from build123d import *

# Parameters (mm, degrees)
ESQUISSE2_R             = 1
ENL_V_MAT_EXTRU_1_DEPTH = 2.6
ESQUISSE3_R             = 1.75
ENL_V_MAT_EXTRU_2_DEPTH = 1.1


with BuildPart() as part:
    # Esquisse1 → Révolution1 (revolve)
    with BuildSketch(Plane(origin=(0, 0, 0), x_dir=(0, 0, -1), z_dir=(1, 0, 0)), mode=Mode.PRIVATE) as r_volution1_sk:
        Polygon((-13.5, 0), (-13.5, 1.15), (-15.6, 1.15), (-15.6, 0), (-20.5, 0), (-20.5, -0.6), (-19.75, -1.6), (-13.1, -1.6), (-13.1, -0.6), (-12.5, -0.6), (-12.5, 0), align=None)
    revolve(r_volution1_sk.sketch.rotate(Axis((0, -40.878639624, 0), (0, 1, 0)), 180), axis=Axis((0, -40.878639624, 0), (0, 1, 0)))  # turned: the seam where the file's is

    # Esquisse2 → Enlèv. mat.-Extru.1 (cut, through all)
    with BuildSketch(Plane(origin=(0, 0, 0), x_dir=(1, 0, 0), z_dir=(0, 1, 0))):
        with Locations(Location((0, -18.4, 0), (0, 0, 270))):  # turned: the seam where the file's is
            Circle(ESQUISSE2_R)
        with Locations(Location((17.4994399, -5.685912696, 0), (0, 0, 270))):  # turned: the seam where the file's is
            Circle(ESQUISSE2_R)
        with Locations(Location((10.815248642, 14.885912696, 0), (0, 0, 270))):  # turned: the seam where the file's is
            Circle(ESQUISSE2_R)
        with Locations(Location((-10.815248642, 14.885912696, 0), (0, 0, 270))):  # turned: the seam where the file's is
            Circle(ESQUISSE2_R)
        with Locations(Location((-17.4994399, -5.685912696, 0), (0, 0, 270))):  # turned: the seam where the file's is
            Circle(ESQUISSE2_R)
    extrude(amount=-ENL_V_MAT_EXTRU_1_DEPTH, mode=Mode.SUBTRACT)

    # Esquisse3 → Enlèv. mat.-Extru.2 (cut)
    with BuildSketch(Plane.XZ.offset(1.6)):
        with Locations(Location((0, 18.4, 0), (0, 0, 270))):  # turned: the seam where the file's is
            Circle(ESQUISSE3_R)
        with Locations(Location((17.4994399, 5.685912696, 0), (0, 0, 270))):  # turned: the seam where the file's is
            Circle(ESQUISSE3_R)
        with Locations(Location((10.815248642, -14.885912696, 0), (0, 0, 270))):  # turned: the seam where the file's is
            Circle(ESQUISSE3_R)
        with Locations(Location((-10.815248642, -14.885912696, 0), (0, 0, 270))):  # turned: the seam where the file's is
            Circle(ESQUISSE3_R)
        with Locations(Location((-17.4994399, 5.685912696, 0), (0, 0, 270))):  # turned: the seam where the file's is
            Circle(ESQUISSE3_R)
    extrude(amount=-ENL_V_MAT_EXTRU_2_DEPTH, mode=Mode.SUBTRACT)


solid = part.part
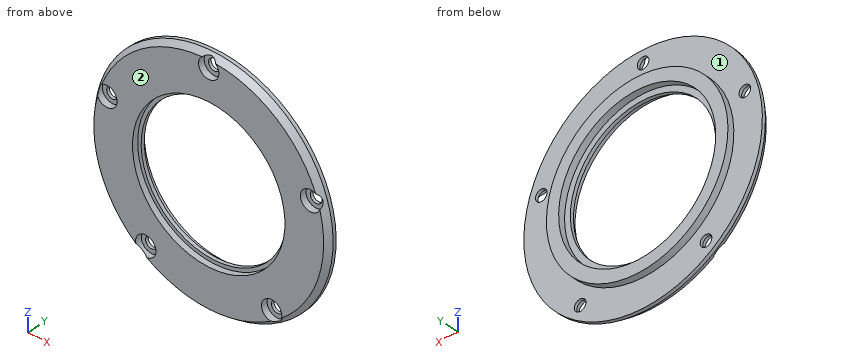
Verification items for the finished model (mm, model axes). Face numbers are marked on the shaded views. A direction names the side the tool comes from. Coordinates: 2 decimals unless noted, no trailing zeros. Order: outer loops, then holes, each group sorted by start corner. A loop starts at its lowest first (then second) coordinate and runs counter-clockwise, first axis right, second up. Notation, with made-up numbers: (-31.5, 63) -> (-10.5, 63) arc R26 cw to (-10.5, 80) -> close; hole circle Ø4 at (64, -26). An arc over 180 degrees is marked (long way). Use CSV: the item, a comma, the result in double quotes. Start each with the question number.
Q1. Section check A-A, the plane z = 0. Record the cut outline in (x, y).
Q2. Depth check by flat-ended pin: P1, Ø3, axis at x = -17.5, z = 5.69, coming from the +Y side; P2, Ø1.5, axis at y = -1, z = 8, coming from the +X side; P3, Ø1, axis at x = 18, z = 5, coming from the -Y side. Enter the tip coordinate at first touch or a pass-through.
Q3. Section check B-B, the plane x = 0. Give the number of separate pieces and of enclosed holes in the cut face, and give its area (3 significant figures).
Q4. Section check C-C, the plane y = 0.65. Record the cut outline in (x, z), and give its area (3 significant figures).
Q5. Tool access check on the marked faces 1 and 2. Record the directions out of +Z, -Z, +X, -X, +Y, -Y that give a thin tool (end or side, any length) a straight path to the whole face; none if there is none.
Q6. Thickness scan on line 1 along Z through (x, y) = (-10, -1.25); line 2 along X through (y, z) = (-0.65, -15.5); line 3 along Y through (x, z) = (5, 17.5). Record the ranges inside material, lowest first.
Returned:
1,outline,"(-20.5, -0.6) -> (-19.75, -1.6) -> (-13.1, -1.6) -> (-13.1, -0.6) -> (-12.5, -0.6) -> (-12.5, 0) -> (-13.5, 0) -> (-13.5, 1.15) -> (-15.6, 1.15) -> (-15.6, 0) -> (-20.5, 0) -> close; (12.5, -0.6) -> (13.1, -0.6) -> (13.1, -1.6) -> (19.75, -1.6) -> (20.5, -0.6) -> (20.5, 0) -> (15.6, 0) -> (15.6, 1.15) -> (13.5, 1.15) -> (13.5, 0) -> (12.5, 0) -> close"
2,P1,"stops at y = 0"
2,P2,"stops at x = 19.13"
2,P3,"stops at y = -0.5"
3,separate pieces,"3"
3,enclosed holes,"0"
3,area,"23.7 mm^2"
4,outline,"circle Ø31.2 at (0, 0); hole circle Ø27 at (0, 0)"
4,area,"192 mm^2"
5,face 1,"+Y"
5,face 2,"+Z, -Z, +X, -X, -Y"
6,line 1,"z = -17.33 to -16.43, -13.34 to -8.46, 8.46 to 17.33"
6,line 2,"x = -13.36 to -12.45, -9.18 to 9.18, 12.45 to 13.36"
6,line 3,"y = -1.6 to 0"
